Part model, mm, in its own coordinate system. Face numbers are marked on the shaded views. A direction names the side the tool comes from. Give positions to 0.01 mm unless a question says otherwise; leave off trailing zeros. Order: outer loops, then holes, each group sorted by start corner. A loop starts at its lowest first (then second) coordinate and runs counter-clockwise, first axis right, second up. Notation, with made-up numbers: M 64.5,78 L 100.5,78 A21 cw 100.5,90 Z; hole C 17.25,4 d11. An arc over 180 degrees is marked long. Answer as a JSON object with one key per item and string values.
from build123d import *

# Parameters (mm, degrees)
SKETCH_1_R          = 26
EXTRUDE_1_DEPTH     = 3
SKETCH_2_R          = 1.4
EXTRUDE_2_DEPTH     = 6
SKETCH_4_R          = 2
EXTRUDE_4_DEPTH     = 2
SKETCH_5_R          = 6
CUT_EXTRUDE_1_DEPTH = 38.25587202
SKETCH_7_R          = 6
SKETCH_7_R_2        = 2.7
EXTRUDE_1_2_DEPTH   = 8
EXTRUDE_START       = 2
SKETCH_8_R          = 3.5
SKETCH_8_R_2        = 2.7
EXTRUDE_2_2_DEPTH   = 2


with BuildPart() as part:
    # 草图1 → Extrude 1 (new body)
    with BuildSketch(Plane.XY):
        Circle(SKETCH_1_R)
    extrude(amount=-EXTRUDE_1_DEPTH)

    # 草图2 → Extrude 2 (add)
    with BuildSketch(Plane.XY):
        with Locations((-21, 0)):
            Circle(SKETCH_2_R)
        with Locations((-10.5, 18.186533479)):
            Circle(SKETCH_2_R)
        with Locations((10.5, 18.186533479)):
            Circle(SKETCH_2_R)
        with Locations((21, 0)):
            Circle(SKETCH_2_R)
        with Locations((10.5, -18.186533479)):
            Circle(SKETCH_2_R)
        with Locations((-10.5, -18.186533479)):
            Circle(SKETCH_2_R)
    extrude(amount=EXTRUDE_2_DEPTH)

    # 草图4 → 凸台-拉伸4 (add)
    with BuildSketch(Plane.XY):
        with Locations((-10.5, 18.186533479)):
            Circle(SKETCH_4_R)
        with Locations((10.5, 18.186533479)):
            Circle(SKETCH_4_R)
        with Locations((21, 0)):
            Circle(SKETCH_4_R)
        with Locations((10.5, -18.186533479)):
            Circle(SKETCH_4_R)
        with Locations((-10.5, -18.186533479)):
            Circle(SKETCH_4_R)
        with Locations((-21, 0)):
            Circle(SKETCH_4_R)
    extrude(amount=EXTRUDE_4_DEPTH)

    # 草图5 → 切除-拉伸1 (cut, through all)
    with BuildSketch(Plane.XY):
        Circle(SKETCH_5_R)
    extrude(amount=-CUT_EXTRUDE_1_DEPTH, mode=Mode.SUBTRACT)

    # 草图7 → Extrude 1 2 (add)
    with BuildSketch(Plane.XY):
        Circle(SKETCH_7_R)
        Circle(SKETCH_7_R_2, mode=Mode.SUBTRACT)
    extrude(amount=-EXTRUDE_1_2_DEPTH)

    # 草图8 → Extrude 2 2 (add)
    with BuildSketch(Plane.XY.offset(EXTRUDE_START)):
        Circle(SKETCH_8_R)
        Circle(SKETCH_8_R_2, mode=Mode.SUBTRACT)
    extrude(amount=-EXTRUDE_2_2_DEPTH)


solid = part.part
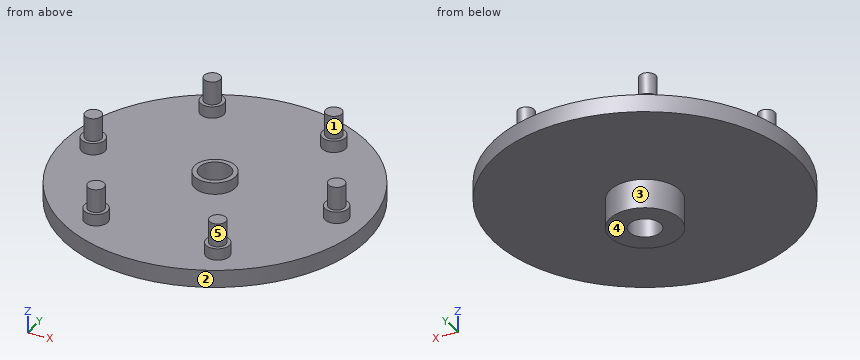
1. Cut at B-B on z = 1. Give the cut face in (x, y).
Worked answers:
{"outline": "C -21,0 d4; C -10.5,-18.19 d4; C -10.5,18.19 d4; C 0,0 d7; C 10.5,-18.19 d4; C 10.5,18.19 d4; C 21,0 d4; hole C 0,0 d5.4"}
2. Pin check, flat tips, straight feed: P1, Ø1.5, axis at y = -2.5, z = -2.5, coming from the -X side; P2, Ø6, axis at y = -19.5, z = -1, coming from the +X side; P3, Ø4, axis at x = -3, z = -4, coming from the -Y side. Stop position of each tip, or through.
Worked answers:
{"P1": "stops at x = -25.94", "P2": "stops at x = 20.09", "P3": "stops at y = -25.97"}
3. Which spindle directions (+Z, -Z, +X, -X, +Y, -Y) get a long thin tool onto all of the face, cutting with end or side? Do the marked faces 1 and 2. Say none if no direction does.
Worked answers:
{"face 1": "+Z", "face 2": "+Z, -Z"}
4. Cut at D-D on x = 21. Give the cut face in (y, z), plus the area to 3 significant figures.
Worked answers:
{"outline": "M -15.33,-3 L 15.33,-3 L 15.33,0 L 2,0 L 2,2 L 1.4,2 L 1.4,6 L -1.4,6 L -1.4,2 L -2,2 L -2,0 L -15.33,0 Z", "area": "111 mm^2"}
5. Cut at C-C on z = -5. Give the cut face in (x, y).
Worked answers:
{"outline": "C 0,0 d12; hole C 0,0 d5.4"}
6. Two-plate mould, pull along X, no slides. Class the marked faces 3, 4 and 5: +X half, -X half, draft (parallel to the pull), parting line (faces both ways), or undercut.
Worked answers:
{"face 3": "parting line", "face 4": "draft", "face 5": "undercut"}
7. Probe line 1 along Y through (x, z) = (0, -4); line 2 along Y through (x, z) = (0, -2); line 3 along X through (y, z) = (18, 5.25). List the from-to ranges inside material, lowest first.
Worked answers:
{"line 1": "y = -6 to -2.7, 2.7 to 6", "line 2": "y = -26 to -2.7, 2.7 to 26", "line 3": "x = -11.89 to -9.11, 9.11 to 11.89"}
8. Cut at A-A on x = 0. Give the cut face in (y, z), plus the area to 3 significant figures.
Worked answers:
{"outline": "M -26,-3 L -6,-3 L -6,-8 L -2.7,-8 L -2.7,2 L -3.5,2 L -3.5,0 L -26,0 Z; M 2.7,-8 L 6,-8 L 6,-3 L 26,-3 L 26,0 L 3.5,0 L 3.5,2 L 2.7,2 Z", "area": "176 mm^2"}
